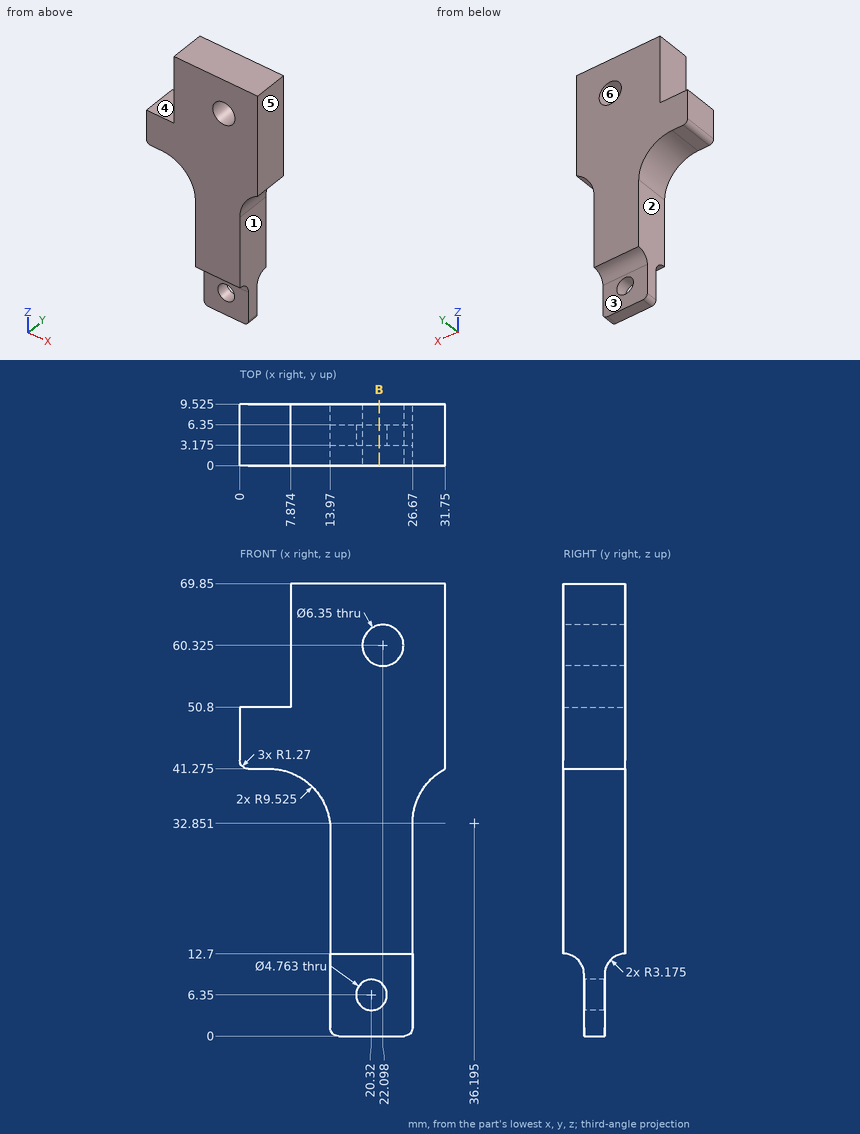
Verification items for this drawing (mm, ordinates from the low corner). A direction names the side the tool comes from. Round coordinates to 2 decimals unless told otherwise and drop trailing zeros. Use one line per item in the form item = value.
1. Go/stop test with flat-tipped pins: pin 1 (4 mm diameter, centred on y = 4.5, z = 15.5, fed in from -X); pin 2 (2.5 mm diameter, centred on x = 6, y = 3.5, fed in from +Z); pin 3 (3.5 mm diameter, centred on x = 3, y = 5.5, fed in from -Z). Record where each tip stops, or that it passes through.
Working result:
pin_1 = 13.97
pin_2 = 50.8
pin_3 = 41.27
2. Mould release check, pull along Z, two halves, no side actions. Record for the marked faces 4, 5 and 6: pulls with the +Z half, pulls with the -Z half, needs draft (parallel to the pull), parting line crosses it, or undercut.
Working result:
face_4 = pulls with the +Z half
face_5 = needs draft
face_6 = undercut
3. Scan lines: line 1 along X through (y, z) = (5.75, 6.35); line 2 along X through (y, z) = (6.75, 23.5); line 3 along Z through (x, y) = (4, 5.5) (1 decimal). Record each from-to range of solid material in increasing order. Write a range as from..to.
Working result:
line_1 = 13.97..17.94, 22.7..26.67
line_2 = 13.97..26.67
line_3 = 41.3..50.8
4. Set-up check for the marked faces 1, 2 and 3: record each of +Z, -Z, +X, -X, +Y, -Y from which the full face is reachable in a straight line by a thin tool's end or side.
Working result:
face_1 = -Z, +X, +Y, -Y
face_2 = -Z, -X, +Y, -Y
face_3 = -Z, +X, -X, +Y
5. Cross-section at B-B, the plane x = 21.5. Count the separate pieces of the cut face and the enclosed holes in it.
Working result:
separate_pieces = 3
enclosed_holes = 0
